Build history of the part. All positions in model axes, mm. A direction names the side the tool comes from. Coordinates: 2 decimals unless noted, no trailing zeros. Loops run counter-clockwise (first coordinate to the right, second up) from the corner with the lowest first, then second, coordinate; pieces in that order, holes last. Notation, with made-up numbers: (41, 2) - (46, 2) arc R27 ccw to (46, 29) - close; hole circle Ø1 at (-35, 56). An arc over 180 degrees is marked (long way). One line per item, written item: value.
```python
from build123d import *

# Parameters (mm, degrees)
BOSS_EXTRUDE2_DEPTH = 1.5
BOSS_EXTRUDE3_DEPTH = 1
FILLET1_R           = 2
CUT_EXTRUDE1_START  = -0.5
CUT_EXTRUDE1_DEPTH  = 0.5
FILLET2_R           = 2


with BuildPart() as part:
    # Sketch1 → Boss-Extrude2 (new body)
    with BuildSketch(Plane.XY):
        Polygon((-50, -67.5), (0, -67.5), (50, -67.5), (50, 67.5), (0, 67.5), (-50, 67.5), align=None)
        Polygon((28, -65), (0, -65), (-28, -65), (-32, -65), (-32, 4), (32, 4), (32, -65), align=None, mode=Mode.SUBTRACT)
        Polygon((-17, 64.5), (0, 64.5), (17, 64.5), (17, 49.5), (17, 21.5), (17, 6.5), (12, 6.5), (0, 6.5), (-12, 6.5), (-17, 6.5), align=None, mode=Mode.SUBTRACT)
    extrude(amount=BOSS_EXTRUDE2_DEPTH)

    # Sketch1_5 → Boss-Extrude3 (add)
    with BuildSketch(Plane.XY):
        Polygon((17, 64.5), (-17, 64.5), (-17, 6.5), (-12, 6.5), (-12, 11.5), (12, 11.5), (12, 6.5), (17, 6.5), (17, 21.5), (-8, 21.5), (-8, 49.5), (17, 49.5), align=None)
        Polygon((-28, -57), (0, -57), (28, -57), (28, -65), (32, -65), (32, 4), (-32, 4), (-32, -65), (-28, -65), align=None)
    extrude(amount=BOSS_EXTRUDE3_DEPTH)

    # Fillet1
    fillet1_edges = [part.edges().sort_by_distance(p)[0] for p in [
        (-50, 67.5, 0.75),
        (50, 67.5, 0.75),
        (50, -67.5, 0.75),
        (-50, -67.5, 0.75),
    ]]
    fillet(fillet1_edges, radius=FILLET1_R)

    # Sketch2 → Cut-Extrude1 (cut)
    with BuildSketch(Plane(origin=(0, 0, 0), x_dir=(-1, 0, 0), z_dir=(0, 0, -1)).offset(CUT_EXTRUDE1_START)):
        with BuildLine():
            Line((-49, -66.5), (-49, 66.5))
            Line((-49, 66.5), (0, 66.5))
            Line((0, 66.5), (0, 67.5))
            Line((0, 67.5), (-48, 67.5))
            ThreePointArc((-48, 67.5), (-49.414213562, 66.914213562), (-50, 65.5))
            Line((-50, 65.5), (-50, -65.5))
            ThreePointArc((-50, -65.5), (-49.414213562, -66.914213562), (-48, -67.5))
            Line((-48, -67.5), (0, -67.5))
            Line((0, -67.5), (0, -66.5))
            Line((0, -66.5), (-49, -66.5))
        make_face()
        with BuildLine():
            Line((0, 67.5), (0, 66.5))
            Line((0, 66.5), (49, 66.5))
            Line((49, 66.5), (49, -66.5))
            Line((49, -66.5), (0, -66.5))
            Line((0, -66.5), (0, -67.5))
            Line((0, -67.5), (48, -67.5))
            ThreePointArc((48, -67.5), (49.414213562, -66.914213562), (50, -65.5))
            Line((50, -65.5), (50, 65.5))
            ThreePointArc((50, 65.5), (49.414213562, 66.914213562), (48, 67.5))
            Line((48, 67.5), (0, 67.5))
        make_face()
    extrude(amount=CUT_EXTRUDE1_DEPTH, mode=Mode.SUBTRACT)

    # Fillet2
    fillet2_edges = [part.edges().sort_by_distance(p)[0] for p in [
        (-49, -66.5, 0.25),
        (-49, 66.5, 0.25),
        (49, 66.5, 0.25),
        (49, -66.5, 0.25),
    ]]
    fillet(fillet2_edges, radius=FILLET2_R)


solid = part.part
```
Item 1: Cut at B-B, the plane z = 1.25. Write the cut outline in (x, y), then the cut area to 3 significant figures.
Check result:
outline: (-50, -65.5) arc R2 ccw to (-48, -67.5) - (48, -67.5) arc R2 ccw to (50, -65.5) - (50, 65.5) arc R2 ccw to (48, 67.5) - (-48, 67.5) arc R2 ccw to (-50, 65.5) - close; hole (-32, -65) - (32, -65) - (32, 4) - (-32, 4) - close; hole (-17, 6.5) - (17, 6.5) - (17, 64.5) - (-17, 64.5) - close
area: 7,110 mm^2
Item 2: Pull direction X, two halves, no side cores. Call faces 3 (the face through (-12, 42, 1)), 4 (the face through (-23, 16, 1.5)): released by +X, released by -X, zero draft, split by the parting line, or undercut.
Check result:
face 3: undercut
face 4: zero draft
Item 3: Cut at C-C, the plane x = 0.5. Write the cut outline in (y, z), then the cut area to 3 significant figures.
Check result:
outline: (-67.5, 0.5) - (-66.5, 0.5) - (-66.5, 0) - (-65, 0) - (-65, 1.5) - (-67.5, 1.5) - close; (-57, 0) - (6.5, 0) - (6.5, 1.5) - (4, 1.5) - (4, 1) - (-57, 1) - close; (11.5, 0) - (21.5, 0) - (21.5, 1) - (11.5, 1) - close; (49.5, 0) - (66.5, 0) - (66.5, 0.5) - (67.5, 0.5) - (67.5, 1.5) - (64.5, 1.5) - (64.5, 1) - (49.5, 1) - close
area: 97.0 mm^2
Item 4: Tool access for faces 1 (the face through (-1, 1, 0)), 2 (the face through (0, -30, 1)): list every direction of +Z, -Z, +X, -X, +Y, -Y with a clear straight run to the whole face (end or side of a thin tool).
Check result:
face 1: -Z, +X, -X, +Y, -Y
face 2: +Z
Item 5: Cut at A-A, the plane x = -21. Write the cut outline in (y, z), then the cut area to 3 significant figures.
Check result:
outline: (-67.5, 0.5) - (-66.5, 0.5) - (-66.5, 0) - (-65, 0) - (-65, 1.5) - (-67.5, 1.5) - close; (-57, 0) - (66.5, 0) - (66.5, 0.5) - (67.5, 0.5) - (67.5, 1.5) - (4, 1.5) - (4, 1) - (-57, 1) - close
area: 159 mm^2
Item 6: Drop a flat-ended pin along its axis: P1, Ø17, axis at x = -5, y = 23, coming from the +Z side. Give the stop position or say it passes through.
Check result:
P1: stops at z = 1
Item 7: Probe probe 1 along Y at (x, z) = (7.5, 1.25); probe 2 along X at (y, z) = (-41.5, 1.05); probe 3 along Y at (x, z) = (-4, 0.8). List the from-to ranges inside material, lowest first. Write a range as from..to.
Check result:
probe 1: y = -67.5..-65, 4..6.5, 64.5..67.5
probe 2: x = -50..-32, 32..50
probe 3: y = -67.5..-65, -57..6.5, 11.5..21.5, 49.5..67.5
Item 8: Cut at D-D, the plane y = -22.5. Write the cut outline in (x, z), then the cut area to 3 significant figures.
Check result:
outline: (-50, 0.5) - (-49, 0.5) - (-49, 0) - (49, 0) - (49, 0.5) - (50, 0.5) - (50, 1.5) - (32, 1.5) - (32, 1) - (-32, 1) - (-32, 1.5) - (-50, 1.5) - close
area: 117 mm^2
